Autodesk Inventor part; units mm, degrees
ref_plane "YZ Plane" through (0, 0, 0) normal (1, 0, 0) x (0, 1, 0)
ref_plane "XZ Plane" through (0, 0, 0) normal (0, 1, 0) x (-1, 0, 0)
ref_plane "XY Plane" through (0, 0, 0) normal (0, 0, 1) x (1, 0, 0)
sketch "Sketch1" plane through (0, 0, 0) normal (0, 0, 1) x (1, 0, 0)
  circle A0 centre (0, 0) radius 2.5
  dimension "Diameter" = 5
extrude "Extrusion1" add sketch "Sketch1" along normal blind 4.9
sketch "Sketch2" plane through (0, 0, 4.9) normal (0, 0, 1) x (1, 0, 0)
  circle A0 centre (0, 0) radius 2.5
extrude "Extrusion2" add sketch "Sketch2" along normal blind 3.1 draft 45
sketch "Sketch3" plane through (0, 0, 8) normal (0, 0, 1) x (1, 0, 0)
  circle A0 centre (0, 0) radius 5.6
  circle A1 centre (0, 0) radius 1.7321 construction
  line L0 (0.725, 1.573) -> (1.7248, 0.1586)
  line L1 (1.7248, 0.1586) -> (0.9997, -1.4144)
  line L2 (0.9997, -1.4144) -> (-0.725, -1.573)
  line L3 (-0.725, -1.573) -> (-1.7248, -0.1586)
  line L4 (-1.7248, -0.1586) -> (-0.9997, 1.4144)
  line L5 (-0.9997, 1.4144) -> (0.725, 1.573)
  dimension "Hex_Width" = 3
extrude "Extrusion3" cut sketch "Sketch3" against normal blind 2 contours L0 L1 L2 L3 L4 L5
thread "Thread1"
chamfer "Chamfer2" distance 0.5 angle 45 1 edges at (-2.5, 0, 0)
fillet "Fillet1" radius 0.1 1 edges at (-5.6, 0, 8)
equation "\"d10\" = Thread_Length"
equation "\"d13\" = Chamfer"
equation "\"Thread_Length\" = 4.9"
equation "\"Length\" = 8"
properties part number "SCREW, FLAT HD, P, 5, M5X0.8X08MM"
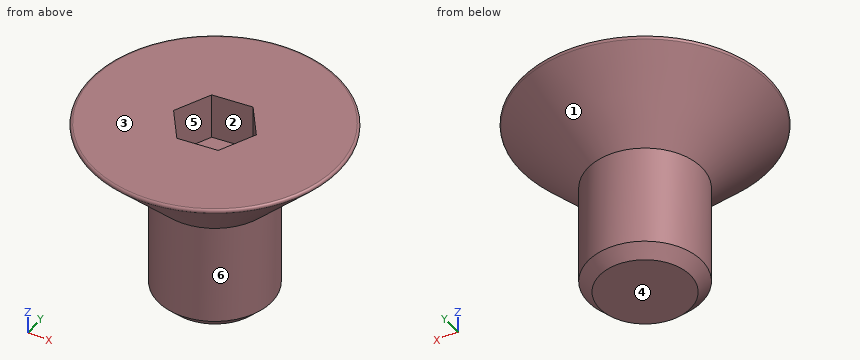
Source: CAD feature listing. Evaluate the final solid. Frame: model axes, mm. Face numbers are marked on the shaded views. A direction names the side the tool comes from. Coordinates: 2 decimals unless noted, no trailing zeros. Loops run counter-clockwise (first coordinate to the right, second up) from the corner with the lowest first, then second, coordinate; pieces in that order, holes last. Notation, with made-up numbers: M 23,0 L 38,0 A8 ccw 38,8 Z; hole C 9.25,1.5 d9. An arc over 180 degrees is marked long. Use CSV: the item, a comma, the result in double quotes.
(1) Line query: line 1 (Z direction, x = 1, y = -1.25); line 2 (Y direction, x = 0, z = 3); line 3 (X direction, y = 1, z = 6.5). Output: solid intervals per line, ascending. Write a range as [from, to].
Answers follow:
line 1,"[0, 6]"
line 2,"[-2.5, 2.5]"
line 3,"[-3.98, -1.19], [1.13, 3.98]"
(2) Cut plane C-C on y = 0. Return loops of the section in (x, z).
Answers follow:
outline,"M -5.43,7.83 L -2.5,4.9 L -2.5,0.5 L -2,0 L 2,0 L 2.5,0.5 L 2.5,4.9 L 5.43,7.83 A0.1 ccw 5.36,8 L 1.65,8 L 1.65,6 L -1.65,6 L -1.65,8 L -5.36,8 A0.1 ccw Z"
(3) Cut plane B-B on x = 0. Return loops of the section in (y, z), and give its area (3 significant figures).
Answers follow:
outline,"M -5.43,7.83 L -2.5,4.9 L -2.5,0.5 L -2,0 L 2,0 L 2.5,0.5 L 2.5,4.9 L 5.43,7.83 A0.1 ccw 5.36,8 L 1.51,8 L 1.51,6 L -1.51,6 L -1.51,8 L -5.36,8 A0.1 ccw Z"
area,"43.3 mm²"
(4) Cut plane D-D on z = 2. Return loops of the section in (x, y).
Answers follow:
outline,"C 0,0 d5"
(5) Reachability of the marked faces 4, 5 and 6 from +Z, -Z, +X, -X, +Y, -Y: full face, straight path, thin tool, end or side. Return the list, or none.
Answers follow:
face 4,"-Z, +X, -X, +Y, -Y"
face 5,"+Z"
face 6,"-Z"
(6) Cut plane A-A on z = 6.25. Return loops of the section in (x, y) (3 decimals).
Answers follow:
outline,"C 0,0 d7.7; hole M -1.725,-0.159 L -0.725,-1.573 L 1,-1.414 L 1.725,0.159 L 0.725,1.573 L -1,1.414 Z"
(7) Draft query along Y for the marked faces 1, 2 and 3. Return one class per face: pulls with the +Y half, pulls with the -Y half, needs draft (parallel to the pull), parting line crosses it, or undercut.
Answers follow:
face 1,"parting line crosses it"
face 2,"undercut"
face 3,"needs draft"
(8) Contact query for flat-ended pins moving along their axis: pin 1 (4 mm diameter, centred on x = 1, z = 1.5, fed in from -Y); pin 2 (2 mm diameter, centred on x = -1.5, y = -4, fed in from -Z); pin 3 (1.5 mm diameter, centred on x = -3.5, z = 6.5, fed in from +Y). Output: stop coordinate, or through.
Answers follow:
pin 1,"y = -2.5"
pin 2,"z = 5.67"
pin 3,"y = 3.58"
